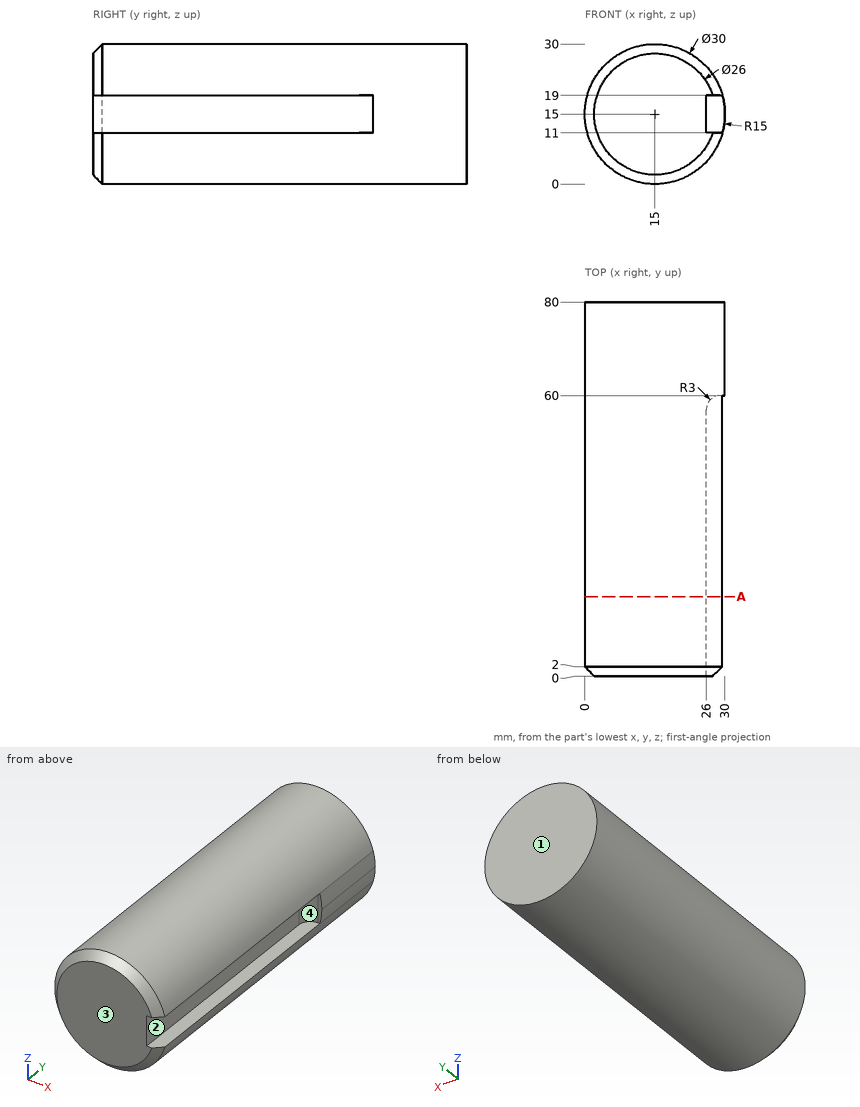
The figure shows three views and two pictorial views of one solid part (mm, origin at its lowest corner). Answer the questions. A direction names the side the tool comes from. Give positions to 0.01 mm unless a question says otherwise; leave off trailing zeros. Loops run counter-clockwise (first coordinate to the right, second up) from the corner with the lowest first, then second, coordinate; pieces in that order, holes last. Notation, with made-up numbers: (60.25, 77.25) - (84.25, 77.25) arc R17 ccw to (84.25, 102.25) - close; hole circle Ø10 at (16.25, 59.25). An arc over 180 degrees is marked (long way). Answer in a Markdown table with one row per item.
(1) Section A-A (y = 17) is taken. Give the vertices of the cut face in (x, z).
Results list:
| item | result |
|---|---|
| outline | (26, 11) - (26, 19) - (29.46, 19) arc R15 ccw (long way) to (29.46, 11) - close |
(2) A tool of negligible diameter and unlimited length cuts with its end or side. For the marked faces 1 and 2, from which of +Z, -Z, +X, -X, +Y, -Y can it reach the whole face along a straight path? Write none if from no direction.
Results list:
| item | result |
|---|---|
| face 1 | +Z, -Z, +X, -X, +Y |
| face 2 | +X, -Y |
(3) For a pull along Z with two mould halves and no side action, classify the marked faces 3 and 4 as pulls with the +Z half, pulls with the -Z half, needs draft (parallel to the pull), parting line crosses it, or undercut.
Results list:
| item | result |
|---|---|
| face 3 | needs draft |
| face 4 | undercut |
(4) Flat-ended cylindrical pins translate along their axes: pin 1 Ø6 at (y, z) = (35.5, 19.5) entering from -X; pin 2 Ø4 at (y, z) = (40, 16) entering from +X; pin 3 Ø1.1 at (x, z) = (29.5, 14.5) entering from -Y. Find the tip coordinate at first contact, or state that the pin passes through.
Results list:
| item | result |
|---|---|
| pin 1 | stops at x = 0.08 |
| pin 2 | stops at x = 26 |
| pin 3 | stops at y = 60 |
(5) Consider L1, parallel to Z at x = 15.5, y = 73.5; L2, parallel to Z at x = 27, y = 35.5; L3, parallel to X at y = 11, z = 14.5. Determine where each line is inside the solid, lowest interval first. Write a range as [from, to].
Results list:
| item | result |
|---|---|
| L1 | z = [0.01, 29.99] |
| L2 | z = [6, 11], [19, 24] |
| L3 | x = [0.01, 26] |
